from build123d import *

# Parameters (mm, degrees)
SKETCH_1_W               = 7.2
SKETCH_1_H               = 24.6
EXTRUDE_1_DEPTH          = 10.8
CUT_EXTRUDE_3_DEPTH      = 7.2
CUT_EXTRUDE_1_DEPTH      = 10.8
EXTRUDE_START            = -3.6
SKETCH_3_R               = 1.1
EXTRUDE_3_DEPTH          = 3.8
CUT_EXTRUDE_2_DEPTH      = 18.963574255
CUT_EXTRUDE_2_DEPTH_BACK = 18.963574255
SKETCH_4_R               = 1.1
CUT_EXTRUDE_4_DEPTH      = 1


with BuildPart() as part:
    # 스케치1 → 보스-돌출1 (new body)
    with BuildSketch(Plane.XY):
        Rectangle(SKETCH_1_W, SKETCH_1_H)
    extrude(amount=EXTRUDE_1_DEPTH)

    # 스케치5 → 컷-돌출3 (cut)
    with BuildSketch(Plane.ZY.offset(3.6)):
        Polygon((0, 12.3), (0, 8.7), (3.6, 12.3), align=None)
    extrude(amount=-CUT_EXTRUDE_3_DEPTH, mode=Mode.SUBTRACT)

    # 스케치2 → 컷-돌출1 (cut)
    with BuildSketch(Plane(origin=(3.6, 0, 0), x_dir=(0, 0, -1), z_dir=(1, 0, 0))):
        Polygon((-10.8, -5.5), (-9, -12.3), (-10.8, -12.3), align=None)
        Polygon((-10.8, 12.3), (-10.8, 10.8), (-9, 12.3), align=None)
        Polygon((-0.9, 7.854415588), (-0.129530009, 8.829530009), (0, 8.7), (0, -5.394280654), (-0.129530009, -5.394280654), (-0.9, -3.854415588), align=None)
        Polygon((-5.55, -12.3), (0, -12.3), (0, -5.5), align=None)
    extrude(amount=-CUT_EXTRUDE_1_DEPTH, mode=Mode.SUBTRACT)

    # 스케치3 → 보스-돌출3 (add)
    with BuildSketch(Plane(origin=(3.6, 0, 0), x_dir=(0, 0, -1), z_dir=(1, 0, 0)).offset(EXTRUDE_START)):
        with BuildLine():
            Line((-3.072792206, 10.772792206), (-5.571079083, 8.27450533))
            Line((-5.571079083, 8.27450533), (-5.571079083, -4.27450533))
            Line((-5.571079083, -4.27450533), (-3.072792206, -6.772792206))
            ThreePointArc((-3.072792206, -6.772792206), (-0.527207794, -6.772792206), (-0.527207794, -4.227207794))
            Line((-0.527207794, -4.227207794), (-1.8, -2.954415588))
            Line((-1.8, -2.954415588), (-1.8, 6.954415588))
            Line((-1.8, 6.954415588), (-0.527207794, 8.227207794))
            ThreePointArc((-0.527207794, 8.227207794), (-0.527207794, 10.772792206), (-3.072792206, 10.772792206))
        make_face()
        with Locations(Location((-1.8, 9.5, 0), (0, 0, 90))):
            Circle(SKETCH_3_R, mode=Mode.SUBTRACT)
        with Locations(Location((-1.8, -5.5, 0), (0, 0, 90))):
            Circle(SKETCH_3_R, mode=Mode.SUBTRACT)
    extrude_3 = extrude(amount=EXTRUDE_3_DEPTH)

    # 스케치4 → 컷-돌출2 (cut, two sides: drawn at the far end of the back side and taken through both)
    with BuildSketch(Plane.ZY.offset(3.6).offset(-CUT_EXTRUDE_2_DEPTH_BACK)):
        with Locations(Location((1.8, 9.5, 0), (0, 0, 90))):
            Circle(SKETCH_4_R)
        with Locations(Location((1.8, -5.5, 0), (0, 0, 90))):
            Circle(SKETCH_4_R)
    extrude(amount=CUT_EXTRUDE_2_DEPTH + CUT_EXTRUDE_2_DEPTH_BACK, mode=Mode.SUBTRACT)

    # 대칭 복사2: 보스-돌출3 across plane
    add(extrude_3.mirror(Plane.ZY))

    # 스케치6 → 컷-돌출4 (cut)
    with BuildSketch(Plane.XY.offset(10.8)):
        with BuildLine():
            Line((1.8, 4.6), (1.8, 0.6))
            ThreePointArc((1.8, 0.6), (0, -1.2), (-1.8, 0.6))
            Line((-1.8, 0.6), (-1.8, 4.6))
            ThreePointArc((-1.8, 4.6), (0, 6.4), (1.8, 4.6))
        make_face()
    extrude(amount=-CUT_EXTRUDE_4_DEPTH, mode=Mode.SUBTRACT)


solid = part.part
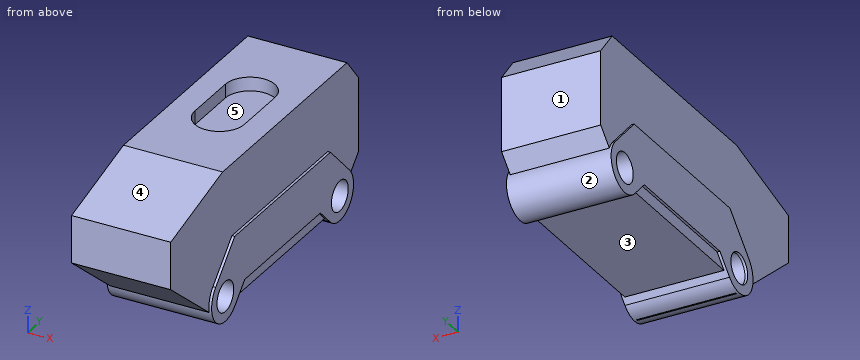
Source: CAD feature listing. Evaluate the final solid. Frame: model axes, mm. Face numbers are marked on the shaded views. A direction names the side the tool comes from. Give positions to 0.01 mm unless a question says otherwise; leave off trailing zeros. Write each loop counter-clockwise with the first axis right and the second up, starting at its lowest first coordinate (ties: lowest second). Pieces come first, ordered by that corner, then holes. Notation, with made-up numbers: M 37,4.25 L 42,4.25 A27 cw 42,39.25 Z; hole C -8.75,-38.5 d4. An arc over 180 degrees is marked long. Return JSON: item names as keys, results as strings. Group by question number.
1) Pull-direction query (Z, two-part tool) for the marked faces 1, 2 and 3; classes: pulls with the +Z half, pulls with the -Z half, needs draft (parallel to the pull), parting line crosses it, or undercut.
2) Set-up query: the marked faces 4 and 5. Return all of +Z, -Z, +X, -X, +Y, -Y with unobstructed straight access to the full face (end or side cutting, diameter ignored); none if empty.
3) Cut plane C-C, the plane z = 6.5. Output: boundary loops of the cut face in (x, y), plus the area to 3 significant figures.
4) Cut plane B-B, the plane y = 9.5. Output: boundary loops of the cut face in (x, z).
5) Cut plane A-A, the plane x = 3. Give the number of separate pieces and of enclosed holes in the cut face, plus the area to 3 significant figures.
6) Pin query (flat end, axial travel): P1, Ø2, axis at x = 1.5, y = 0, coming from the -Z side; P2, Ø3, axis at x = -0.5, y = -3, coming from the -Z side; P3, Ø2, axis at x = -3, z = 4, coming from the -Y side. Return the tip coordinate at first contact, or that it passes through.
7) Material intervals for line 1 along Z through (x, y) = (-1.25, 9.5); line 2 along X through (y, z) = (-2, 8.5); line 3 along Z through (x, y) = (0.75, 1), sorted ascending. Write a range as [from, to].
8) Cut plane D-D, the plane y = -9. Output: boundary loops of the cut face in (x, z), plus the area to 3 significant figures.
Recorded:
{
 "1": {"face 1": "needs draft", "face 2": "undercut", "face 3": "pulls with the -Z half"},
 "2": {"face 4": "+Z, +X, -X, -Y", "face 5": "+Z"},
 "3": {"outline": "M -3.6,-12.3 L 3.6,-12.3 L 3.6,12.3 L -3.6,12.3 Z", "area": "177 mm²"},
 "4": {"outline": "M -3.8,0 L 3.8,0 L 3.8,0.7 L -3.8,0.7 Z; M -3.8,2.9 L 3.8,2.9 L 3.8,4.35 L 3.6,4.35 L 3.6,10.8 L -3.6,10.8 L -3.6,4.35 L -3.8,4.35 Z"},
 "5": {"separate pieces": "1", "enclosed holes": "2", "area": "217 mm²"},
 "6": {"P1": "stops at z = 0.9", "P2": "stops at z = 0.3", "P3": "stops at y = -11.63"},
 "7": {"line 1": "z = [0, 0.7], [2.9, 10.8]", "line 2": "x = [-3.6, 3.6]", "line 3": "z = [0.9, 9.8]"},
 "8": {"outline": "M -3.6,2.86 L 3.6,2.86 L 3.6,9.87 L -3.6,9.87 Z", "area": "50.5 mm²"}
}
